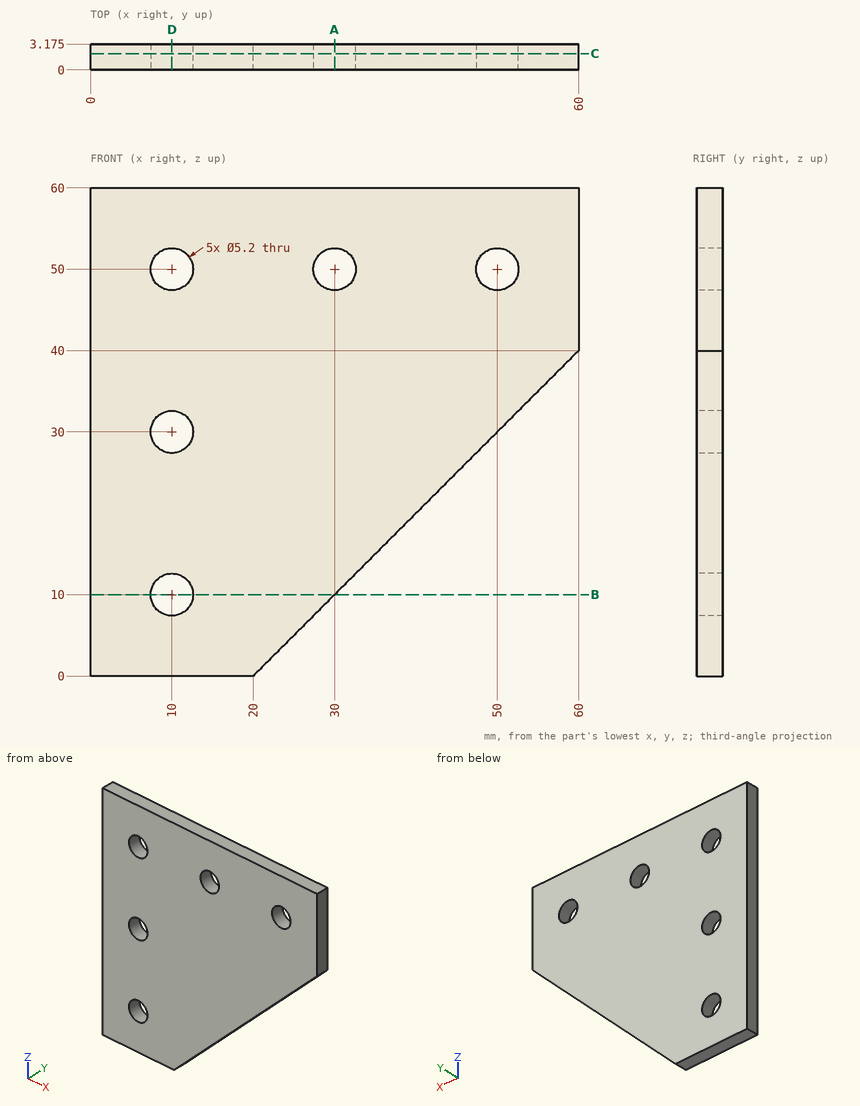
For this review, use the dimensioned drawing (mm, ordinates from the lowest corner) and the shaded views. Give positions to 0.01 mm unless a question says otherwise; leave off trailing zeros. Loops run counter-clockwise (first coordinate to the right, second up) from the corner with the lowest first, then second, coordinate; pieces in that order, holes last. Notation, with made-up numbers: (-19.75, -27.75) -> (-5.75, -27.75) arc R24 ccw to (-5.75, 2.25) -> close; hole circle Ø5 at (77, 39.25). An arc over 180 degrees is marked (long way). One line per question, with ' | ' between items. Start each with the question number.
(1) We need section B-B (z = 10). State the section outline as (x, y) points (3 decimals), and give its area (3 significant figures).
(2) We need section A-A (x = 30). State the section outline as (y, z) points (3 decimals).
(3) We need section C-C (y = 2). State the section outline as (x, z) points, and give its area (3 significant figures).
(4) For line 1 (Z direction, x = 10, y = 2.3); line 2 (X direction, y = 1.55, z = 51); line 3 (X direction, y = 2.9, z = 31.5), list the stretches that pass through material, from the lowest coordinate up.
(5) We need section D-D (x = 10). State the section outline as (y, z) points (3 decimals).
(6) Insertion check: P1, Ø3, axis at x = 30, z = 50, coming from the +Y side. The pin has a flat end and moves straight along its axis. Give the tip position at first contact, or say it passes through.
The answers:
1) outline: (0, 0) -> (7.4, 0) -> (7.4, 3.175) -> (0, 3.175) -> close; (12.6, 0) -> (30, 0) -> (30, 3.175) -> (12.6, 3.175) -> close | area: 78.7 mm^2
2) outline: (0, 10) -> (3.175, 10) -> (3.175, 47.4) -> (0, 47.4) -> close; (0, 52.6) -> (3.175, 52.6) -> (3.175, 60) -> (0, 60) -> close
3) outline: (0, 0) -> (20, 0) -> (60, 40) -> (60, 60) -> (0, 60) -> close; hole circle Ø5.2 at (10, 10); hole circle Ø5.2 at (10, 30); hole circle Ø5.2 at (10, 50); hole circle Ø5.2 at (30, 50); hole circle Ø5.2 at (50, 50) | area: 2,690 mm^2
4) line 1: z = 0 to 7.4, 12.6 to 27.4, 32.6 to 47.4, 52.6 to 60 | line 2: x = 0 to 7.6, 12.4 to 27.6, 32.4 to 47.6, 52.4 to 60 | line 3: x = 0 to 7.88, 12.12 to 51.5
5) outline: (0, 0) -> (3.175, 0) -> (3.175, 7.4) -> (0, 7.4) -> close; (0, 12.6) -> (3.175, 12.6) -> (3.175, 27.4) -> (0, 27.4) -> close; (0, 32.6) -> (3.175, 32.6) -> (3.175, 47.4) -> (0, 47.4) -> close; (0, 52.6) -> (3.175, 52.6) -> (3.175, 60) -> (0, 60) -> close
6) P1: passes through
